Verification items for the finished model (mm, model axes). Coordinates: 2 decimals unless noted, no trailing zeros. Order: outer loops, then holes, each group sorted by start corner. A loop starts at its lowest first (then second) coordinate and runs counter-clockwise, first axis right, second up. Notation, with made-up numbers: M -25,36.25 L 6,36.25 A25 ccw 6,72.25 Z; hole C 50,-11 d11. An arc over 180 degrees is marked long. Return JSON: item names as keys, results as strings. Group by question number.
Q1. Section check A-A, the plane z = 103. Enter the section's corners in (x, y).
Q2. Go/stop test with flat-tipped pins: pin 1 Ø1.5 at (x, y) = (0.5, -0.5) entering from +Z; pin 2 Ø1.5 at (x, y) = (0.5, -2.5) entering from -Z; pin 3 Ø1.2 at (x, z) = (-0.5, 130) entering from -Y; pin 4 Ø4 at (y, z) = (-1.5, 46.5) entering from +X. Record where each tip stops, or that it passes through.
Q3. Thickness scan on probe 1 along Z at (x, y) = (0.25, -0.75); probe 2 along Z at (x, y) = (2.25, -0.75); probe 3 along Z at (x, y) = (-1, 0.25). Record the ranges inside material, lowest first.
from build123d import *

# Parameters (mm, degrees)
EXTRUDE_2_DEPTH     = 140
SKETCH_4_W          = 6
SKETCH_4_H          = 19
CUT_EXTRUDE_1_DEPTH = 1
SKETCH_3_R          = 3
EXTRUDE_4_DEPTH     = 5
CHAMFER_2_SIZE      = 1
FILLET_2_R          = 2
SKETCH_5_W          = 1
SKETCH_5_H          = 102
EXTRUDE_5_DEPTH     = 5
FILLET_3_R          = 1


with BuildPart() as part:
    # 草图2 → 凸台-拉伸2 (new body)
    with BuildSketch(Plane.XY):
        with BuildLine():
            Line((-3, 0), (3, 0))
            Line((3, 0), (3, 1))
            ThreePointArc((3, 1), (0, 4), (-3, 1))
            Line((-3, 1), (-3, 0))
        make_face()
    extrude(amount=EXTRUDE_2_DEPTH)

    # 草图4 → 切除-拉伸1 (cut)
    with BuildSketch(Plane.XZ):
        with Locations((0, 130.5)):
            Rectangle(SKETCH_4_W, SKETCH_4_H)
        with Locations((0, 9.5)):
            Rectangle(SKETCH_4_W, SKETCH_4_H)
    extrude(amount=-CUT_EXTRUDE_1_DEPTH, mode=Mode.SUBTRACT)

    # 草图3 → 凸台-拉伸4 (add)
    with BuildSketch(Plane.XZ.offset(-1)):
        with Locations(Location((0, 131, 0), (0, 0, 180))):
            Circle(SKETCH_3_R)
        with Locations(Location((0, 9, 0), (0, 0, 180))):
            Circle(SKETCH_3_R)
    extrude(amount=EXTRUDE_4_DEPTH)

    # 倒角2
    chamfer_2_edges = [part.edges().sort_by_distance(p)[0] for p in [
        (3, -4, 131),
        (3, -4, 9),
    ]]
    chamfer(chamfer_2_edges, length=CHAMFER_2_SIZE)

    # 圆角2
    fillet_2_edges = [part.edges().sort_by_distance(p)[0] for p in [
        (0, 4, 140),
        (0, 4, 0),
    ]]
    fillet(fillet_2_edges, radius=FILLET_2_R)

    # 草图5 → 凸台-拉伸5 (add)
    with BuildSketch(Plane.XZ):
        with Locations((0, 70)):
            Rectangle(SKETCH_5_W, SKETCH_5_H)
    extrude(amount=EXTRUDE_5_DEPTH)

    # 圆角3
    fillet_3_edges = [part.edges().sort_by_distance(p)[0] for p in [
        (0, -5, 19),
        (0, -5, 121),
    ]]
    fillet(fillet_3_edges, radius=FILLET_3_R)


solid = part.part
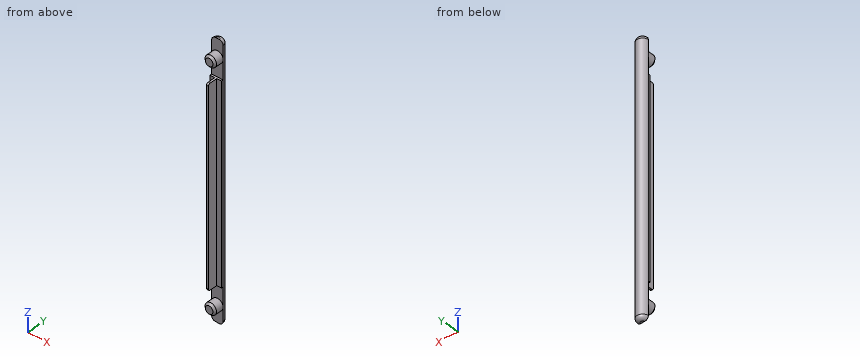
Numbers:
{
 "1": {"outline": "M -3,0 L -0.5,0 L -0.5,-5 L 0.5,-5 L 0.5,0 L 3,0 L 3,1 A3 ccw -3,1 Z"},
 "2": {"pin 1": "stops at z = 134", "pin 2": "stops at z = 6", "pin 3": "stops at y = -4", "pin 4": "stops at x = 3"},
 "3": {"probe 1": "z = 6.01 to 11.99, 19 to 121, 128.01 to 133.99", "probe 2": "z = 7.02 to 10.98, 129.02 to 132.98", "probe 3": "z = 6.17 to 11.83, 19 to 121, 128.17 to 133.83"}
}
